```python
from build123d import *

# Parameters (mm, degrees)
EXTRUDE_1_DEPTH     = 10
FILLET_1_R          = 12
FILLET_2_R          = 6
EXTRUDE_2_DEPTH     = 25
EXTRUDE_3_DEPTH     = 35
SKETCH_2_4_W        = 70
SKETCH_2_4_H        = 25
CUT_EXTRUDE_1_DEPTH = 35
FILLET_3_R          = 6
FILLET_4_R          = 12
FILLET_5_R          = 3
CUT_EXTRUDE_START   = -35
CUT_EXTRUDE_2_DEPTH = 35
EXTRUDE_START       = 35
EXTRUDE_4_DEPTH     = 10
EXTRUDE_START_2     = 32
SKETCH_6_4_R        = 19
SKETCH_6_4_R_2      = 10
EXTRUDE_5_DEPTH     = 16
SKETCH_7_R          = 5
CUT_EXTRUDE_3_DEPTH = 144.506097431


with BuildPart() as part:
    # 草图1 → 凸台-拉伸1 (new body)
    with BuildSketch(Plane(origin=(0, 0, 0), x_dir=(1, 0, 0), z_dir=(0, 1, 0))):
        Polygon((45, 0), (45, 40), (69, 40), (69, 78), (75, 78), (75, 88), (-75, 88), (-75, 78), (-69, 78), (-69, 40), (-45, 40), (-45, 0), align=None)
    extrude(amount=-EXTRUDE_1_DEPTH)

    # 圆角1
    fillet_1_edges = [part.edges().sort_by_distance(p)[0] for p in [
        (-45, -5, -40),
        (45, -5, -40),
    ]]
    fillet(fillet_1_edges, radius=FILLET_1_R)

    # 圆角2
    fillet_2_edges = [part.edges().sort_by_distance(p)[0] for p in [
        (69, -5, -78),
        (-69, -5, -78),
    ]]
    fillet(fillet_2_edges, radius=FILLET_2_R - 0.0001)  # a hair under: the kernel refuses the full size

    # 草图2 → 凸台-拉伸2 (add)
    with BuildSketch(Plane(origin=(0, 0, 0), x_dir=(1, 0, 0), z_dir=(0, 1, 0))):
        with BuildLine():
            Line((-25, 53), (-25, 28))
            ThreePointArc((-25, 28), (-17.67766953, 45.67766953), (0, 53))
            Line((0, 53), (0, 63))
            Line((0, 63), (-35, 63))
            Line((-35, 63), (-35, 88))
            Line((-35, 88), (-75, 88))
            Line((-75, 88), (-75, 78))
            Line((-75, 78), (-45, 78))
            Line((-45, 78), (-45, 53))
            Line((-45, 53), (-25, 53))
        make_face()
        with BuildLine():
            ThreePointArc((0, 53), (17.67766953, 45.67766953), (25, 28))
            Line((25, 28), (25, 53))
            Line((25, 53), (45, 53))
            Line((45, 53), (45, 78))
            Line((45, 78), (75, 78))
            Line((75, 78), (75, 88))
            Line((75, 88), (35, 88))
            Line((35, 88), (35, 63))
            Line((35, 63), (0, 63))
            Line((0, 63), (0, 53))
        make_face()
    extrude(amount=EXTRUDE_2_DEPTH)

    # 草图2<3> → 凸台-拉伸3 (add)
    with BuildSketch(Plane(origin=(0, 0, 0), x_dir=(1, 0, 0), z_dir=(0, 1, 0))):
        with BuildLine():
            ThreePointArc((-25, 28), (-17.67766953, 10.32233047), (0, 3))
            Line((0, 3), (0, 12))
            ThreePointArc((0, 12), (-16, 28), (0, 44))
            Line((0, 44), (0, 53))
            ThreePointArc((0, 53), (-17.67766953, 45.67766953), (-25, 28))
        make_face()
        with BuildLine():
            Line((0, 12), (0, 3))
            ThreePointArc((0, 3), (17.67766953, 10.32233047), (25, 28))
            ThreePointArc((25, 28), (17.67766953, 45.67766953), (0, 53))
            Line((0, 53), (0, 44))
            ThreePointArc((0, 44), (11.313708499, 39.313708499), (16, 28))
            ThreePointArc((16, 28), (11.313708499, 16.686291501), (0, 12))
        make_face()
    extrude(amount=EXTRUDE_3_DEPTH)

    # 草图2<4> → 切除-拉伸1 (cut)
    with BuildSketch(Plane(origin=(0, 0, 0), x_dir=(1, 0, 0), z_dir=(0, 1, 0))):
        with Locations((0, 75.5)):
            Rectangle(SKETCH_2_4_W, SKETCH_2_4_H)
    extrude(amount=-CUT_EXTRUDE_1_DEPTH, mode=Mode.SUBTRACT)

    # 圆角3
    fillet_3_edges = [part.edges().sort_by_distance(p)[0] for p in [
        (45, 12.5, -78),
        (-45, 12.5, -78),
    ]]
    fillet(fillet_3_edges, radius=FILLET_3_R)

    # 圆角4
    fillet_4_edges = [part.edges().sort_by_distance(p)[0] for p in [
        (45, 12.5, -53),
        (-45, 12.5, -53),
    ]]
    fillet(fillet_4_edges, radius=FILLET_4_R)

    # 圆角5
    fillet_5_edges = [part.edges().sort_by_distance(p)[0] for p in [
        (35, 7.5, -63),
        (-35, 7.5, -63),
    ]]
    fillet(fillet_5_edges, radius=FILLET_5_R)

    # 草图2<5> → 切除-拉伸2 (cut)
    with BuildSketch(Plane(origin=(0, 0, 0), x_dir=(1, 0, 0), z_dir=(0, 1, 0)).offset(CUT_EXTRUDE_START)):
        with BuildLine():
            ThreePointArc((0, 44), (-16, 28), (0, 12))
            Line((0, 12), (0, 44))
        make_face()
        with BuildLine():
            Line((0, 44), (0, 12))
            ThreePointArc((0, 12), (11.313708499, 16.686291501), (16, 28))
            ThreePointArc((16, 28), (11.313708499, 39.313708499), (0, 44))
        make_face()
    extrude(amount=CUT_EXTRUDE_2_DEPTH, mode=Mode.SUBTRACT)

    # 草图6 → 凸台-拉伸4 (add)
    with BuildSketch(Plane(origin=(0, 0, 0), x_dir=(0, 0, -1), z_dir=(1, 0, 0)).offset(EXTRUDE_START)):
        with BuildLine():
            Line((0, -10), (9.228717941, -68.939212458))
            ThreePointArc((9.228717941, -68.939212458), (26.525951004, -47.057265785), (47, -66))
            ThreePointArc((47, -66), (46.868026287, -68.235527685), (46.473938523, -70.439999487))
            Line((46.473938523, -70.439999487), (56.431805566, -29.007331733))
            Line((56.431805566, -29.007331733), (61, -10))
            Line((61, -10), (0, -10))
        make_face()
    extrude_4 = extrude(amount=EXTRUDE_4_DEPTH)

    # 草图6<4> → 凸台-拉伸5 (add)
    with BuildSketch(Plane(origin=(0, 0, 0), x_dir=(0, 0, -1), z_dir=(1, 0, 0)).offset(EXTRUDE_START_2)):
        with Locations((28, -66)):
            Circle(SKETCH_6_4_R)
        with Locations((28, -66)):
            Circle(SKETCH_6_4_R_2, mode=Mode.SUBTRACT)
    extrude_5 = extrude(amount=EXTRUDE_5_DEPTH)

    # 镜向1: 凸台-拉伸4, 凸台-拉伸5 across plane
    add(extrude_4.mirror(Plane(origin=(0, 0, 0), x_dir=(0, 0, 1), z_dir=(1, 0, 0))))
    add(extrude_5.mirror(Plane(origin=(0, 0, 0), x_dir=(0, 0, 1), z_dir=(1, 0, 0))))

    # 草图7 → 切除-拉伸3 (cut, through all)
    with BuildSketch(Plane.XY):
        with Locations((-63, 13)):
            Circle(SKETCH_7_R)
    cut_extrude_3 = extrude(amount=-CUT_EXTRUDE_3_DEPTH, mode=Mode.SUBTRACT)

    # 镜向2: 切除-拉伸3 across plane
    add(cut_extrude_3.mirror(Plane(origin=(0, 0, 0), x_dir=(0, 0, 1), z_dir=(1, 0, 0))), mode=Mode.SUBTRACT)


solid = part.part
```
CAD build for the part. Positions are in the model's coordinates, mm. A direction names the side the tool comes from. Coordinates: 2 decimals unless noted, no trailing zeros. Write each loop counter-clockwise with the first axis right and the second up, starting at its lowest first coordinate (ties: lowest second). Pieces come first, ordered by that corner, then holes.
(1) Cut at C-C, the plane x = -63. List the corners of the cut face in (y, z).
(2) Drill centre lines: probe 1 along Y at (x, z) = (40, -28); probe 2 along X at (y, z) = (-20, -5.5); probe 3 along X at (y, z) = (-53, -30). Where is each one in solid material? Low to high.
(3) Two-plate mould, pull along X, no slides. Class faces 4 (the face through (-58, 11, -78)), 5 (the face through (0, 7, -63)), 6 (the face through (25, 12, -40)): +X half, -X half, draft (parallel to the pull), parting line (faces both ways), or undercut.
(4) Cut at B-B, the plane y = 13. Count the separate pieces of the cut face and the enclosed holes in it, and give its area (4 significant figures).
(5) 3-axis set-ups, long thin cutter, end or side, ignore diameter. For faces 1 (the face through (-45, 12, -69)), 2 (the face through (32, -74, -36)), 3 (the face through (68, 11, -78)): which of +Z, -Z, +X, -X, +Y, -Y reach the whole face in a straight line?
(6) Flat gauge pins, fed straight in: pin 1 (23.5 mm diameter, centred on x = 30, z = -57, fed in from +Y); pin 2 (1 mm diameter, centred on y = -28.5, z = -33.5, fed in from -X); pin 3 (6 mm diameter, centred on x = -55.5, z = -36, fed in from -Y); pin 4 (19 mm diameter, centred on y = -66.5, z = -20.5, fed in from +X). Where does each tip first touch, or does it go through?
(7) Cut at A-A, the plane z = -68. List the corners of the cut face in (x, y), and give its area (3 significant figures).
Geometry says:
1. outline: (-10, -88) - (8, -88) - (8, -78) - (0, -78) - (0, -40) - (-10, -40) - close; (18, -88) - (25, -88) - (25, -78) - (18, -78) - close
2. probe 1: y = -85 to -76, -56 to 0
2. probe 2: x = -45 to -35, 35 to 45
2. probe 3: x = -48 to -32, 32 to 48
3. face 4: draft
3. face 5: undercut
3. face 6: +X half
4. separate pieces: 3
4. enclosed holes: 1
4. area: 3,185 mm2
5. face 1: +Z, -X, +Y
5. face 2: +Z, -Z, -Y
5. face 3: +Z, +X, +Y
6. pin 1: stops at y = 25
6. pin 2: stops at x = -45
6. pin 3: passes through
6. pin 4: stops at x = 48
7. outline: (-69, -10) - (-35, -10) - (-35, 25) - (-45, 25) - (-45, 0) - (-69, 0) - close; (35, -10) - (69, -10) - (69, 0) - (45, 0) - (45, 25) - (35, 25) - close
7. area: 1,180 mm2
